Input: part model. Units: mm. Frame: model coordinates. Face numbers are marked on the shaded views. A direction names the side the tool comes from. Coordinates: 2 decimals unless noted, no trailing zeros. Write each loop counter-clockwise with the first axis right and the second up, starting at its lowest first coordinate (ties: lowest second). Pieces come first, ordered by that corner, then holes. Notation, with made-up numbers: (1, 66.25) - (22, 66.25) arc R23 ccw to (22, 77.25) - close; hole circle Ø4 at (-26.75, 67). An arc over 180 degrees is marked (long way). Put each result on its own line as item: value. Start each with the question number.
1. Line query: line 1 (X direction, y = 3.5, z = 6.25); line 2 (X direction, y = -4.5, z = 8.5); line 3 (Y direction, x = 4.5, z = 3.5). Output: solid intervals per line, ascending.
2. Cut plane A-A, the plane y = -2.75. Return loops of the section in (x, z), and give its area (3 significant figures).
3. Pin query (flat end, axial travel): pin 1 (4 mm diameter, centred on y = -4, z = 3, fed in from -X); pin 2 (3 mm diameter, centred on y = 1, z = 5.5, fed in from +X); pin 3 (5 mm diameter, centred on y = -2.5, z = 3, fed in from -X). Return the tip coordinate at first contact, or that it passes through.
4. Pull-direction query (Y, two-part tool) for the marked faces 1, 2, 3 and 4; classes: released by +Y, released by -Y, zero draft, split by the parting line, or undercut.
5. Access query for the marked faces 5, 6 and 7. Directions: +Z, -Z, +X, -X, +Y, -Y. A direction counts if a zero-diameter tool reaches every point of the face in a straight line with its end or side. Return the directions, or none.
from build123d import *

# Parameters (mm, degrees)
SKETCH1_R           = 4.25
BOSS_EXTRUDE1_DEPTH = 10
BOSS_EXTRUDE2_DEPTH = 10
CIRPATTERN1_COUNT   = 11
SKETCH5_R           = 3
CUT_EXTRUDE1_DEPTH  = 10
FILLET1_R           = 0.4
FILLET2_R           = 0.1


with BuildPart() as part:
    # Sketch1 → Boss-Extrude1 (new body)
    with BuildSketch(Plane.XY):
        Circle(SKETCH1_R)
    extrude(amount=BOSS_EXTRUDE1_DEPTH)

    # Sketch3 → Boss-Extrude2 (add)
    with BuildSketch(Plane.XY):
        Polygon((0, 6.174026833), (0.527734359, 5.897416886), (0.8, 4.174026833), (-0.8, 4.174026833), (-0.522537345, 5.897416886), align=None)
    boss_extrude2 = extrude(amount=BOSS_EXTRUDE2_DEPTH)

    # CirPattern1: Boss-Extrude2 ×11 about axis
    cirpattern1_axis = Axis((0, 0, 0), (0, 0, 1))
    for i in range(1, CIRPATTERN1_COUNT):
        add(boss_extrude2.rotate(cirpattern1_axis, i * 360 / CIRPATTERN1_COUNT))

    # Sketch5 → Cut-Extrude1 (cut)
    with BuildSketch(Plane.XY):
        Circle(SKETCH5_R)
    extrude(amount=CUT_EXTRUDE1_DEPTH, mode=Mode.SUBTRACT)

    # Fillet1
    fillet1_edges = [part.edges().sort_by_distance(p)[0] for p in [
        (1.943553631, -3.779563372, 5),
        (0.408364873, -4.230335463, 5),
        (3.678407589, -2.128806616, 5),
        (2.630630415, -3.338005935, 5),
        (4.245393129, 0.1978312, 5),
        (4.017689387, -1.385883107, 5),
        (3.464496346, 2.461659007, 5),
        (4.129160367, 1.006247815, 5),
        (1.583646453, 3.943927473, 5),
        (2.929652105, 3.078902165, 5),
        (-2.929652105, 3.078902165, 5),
        (-1.583646453, 3.943927473, 5),
        (-4.129160367, 1.006247815, 5),
        (-3.464496346, 2.461659007, 5),
        (-4.017689387, -1.385883107, 5),
        (-4.245393129, 0.1978312, 5),
        (-2.630630415, -3.338005935, 5),
        (-3.678407589, -2.128806616, 5),
        (-0.408364873, -4.230335463, 5),
        (-1.943553631, -3.779563372, 5),
        (-0.8, 4.174026833, 5),
        (0.8, 4.174026833, 5),
    ]]
    fillet(fillet1_edges, radius=FILLET1_R)

    # Fillet2
    fillet2_edges = [part.edges().sort_by_distance(p)[0] for p in [
        (0.527734359, 5.897416886, 5),
        (2.162865249, -5.511314283, 5),
        (1.155136929, -5.807210015, 5),
        (4.799159491, -3.467079374, 5),
        (4.111377792, -4.260821767, 5),
        (5.911754503, -0.322071262, 5),
        (5.762285256, -1.361652714, 5),
        (5.147409232, 2.9251922, 5),
        (5.583707865, 1.969831455, 5),
        (2.748797899, 5.243727807, 5),
        (3.63234268, 4.675908055, 5),
        (-3.627970674, 4.678717773, 5),
        (-2.744425893, 5.246537525, 5),
        (-5.581548948, 1.974558825, 5),
        (-5.145250314, 2.92991957, 5),
        (-5.763024868, -1.356508599, 5),
        (-5.912494116, -0.316927147, 5),
        (-4.666018151, -4.043127743, 5),
        (-4.802562811, -3.463151734, 5),
        (-1.160123427, -5.805745847, 5),
        (-2.167851747, -5.509850115, 5),
        (-0.522537345, 5.897416886, 5),
    ]]
    fillet(fillet2_edges, radius=FILLET2_R)


solid = part.part
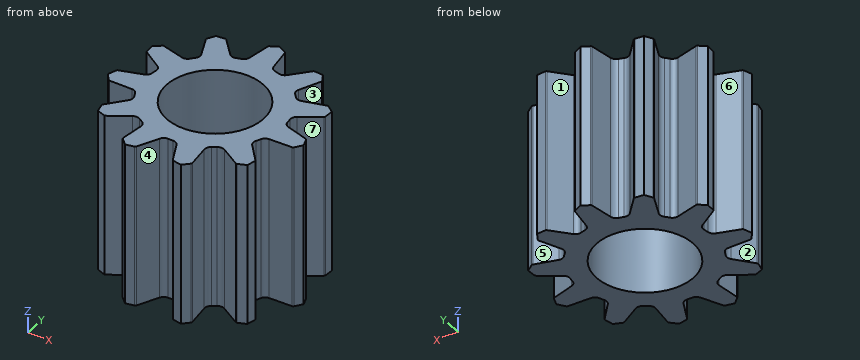
Report:
1. line 1: x = -3.11 to 3.11
1. line 2: x = -2.04 to -0.54, 0.54 to 2.03
1. line 3: y = -4.11 to -3.11, -1.38 to 0.12, 1.25 to 2.75
2. outline: (-4.2, 0) - (-1.2, 0) - (-1.2, 10) - (-4.2, 10) - close; (1.2, 0) - (4.2, 0) - (4.2, 10) - (1.2, 10) - close
2. area: 60.0 mm^2
3. pin 1: stops at x = -4.79
3. pin 2: stops at x = 5.98
3. pin 3: stops at x = -6.11
4. face 1: released by +Y
4. face 2: undercut
4. face 3: undercut
4. face 4: released by -Y
5. face 5: +Z, -Z, +Y
5. face 6: +Z, -Z, -X
5. face 7: +Z, -Z, +X
